Design review of the part shown in the three views and the two pictorial views. Dimensions are in mm from the part's minimum x, y and z. Give positions to 0.01 mm unless a question says otherwise; leave off trailing zeros. Order: outer loops, then holes, each group sorted by start corner. A loop starts at its lowest first (then second) coordinate and runs counter-clockwise, first axis right, second up. Notation, with made-up numbers: (8.5, -24.75) - (65.5, -24.75) arc R29 ccw to (65.5, 7.25) - close; hole circle Ø6 at (22.25, -3). An arc over 180 degrees is marked (long way). Put each result on its own line as item: value. Start each with the question number.
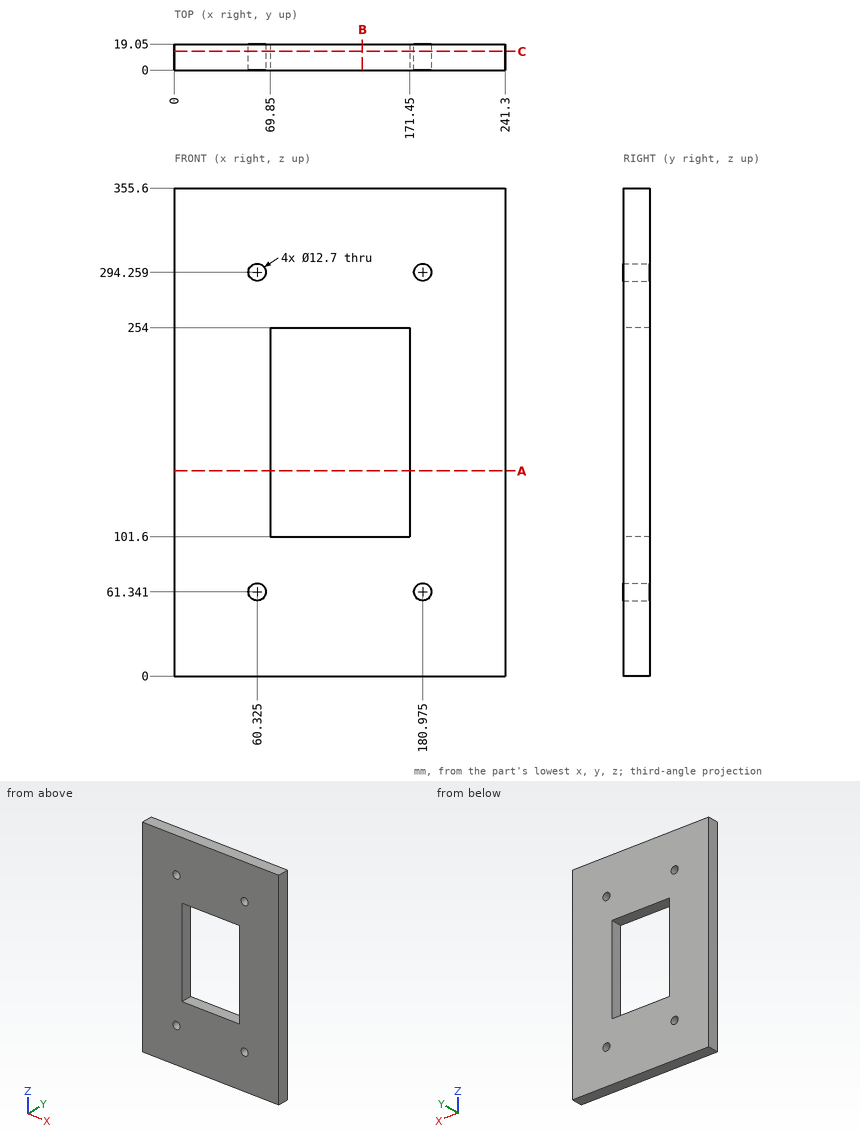
1. Add section A-A, the plane z = 149.5. Give the boundary of the cut face in (x, y).
2. Add section B-B, the plane x = 137. Give the boundary of the cut face in (y, z), then the cut area to 3 significant figures.
3. Add section C-C, the plane y = 13.75. Give the boundary of the cut face in (x, z) (3 decimals).
4. Wall thickness on line 1 (Z direction, x = 97, y = 14.5); line 2 (Z direction, x = 180, y = 12.5); line 3 (X direction, y = 7.25, z = 212.5): over which ranges is each line inside the solid? List them lowest first. Write a range as from..to.
Found:
1. outline: (0, 0) - (69.85, 0) - (69.85, 19.05) - (0, 19.05) - close; (171.45, 0) - (241.3, 0) - (241.3, 19.05) - (171.45, 19.05) - close
2. outline: (0, 0) - (19.05, 0) - (19.05, 101.6) - (0, 101.6) - close; (0, 254) - (19.05, 254) - (19.05, 355.6) - (0, 355.6) - close
2. area: 3,870 mm^2
3. outline: (0, 0) - (241.3, 0) - (241.3, 355.6) - (0, 355.6) - close; hole circle Ø12.7 at (60.325, 61.341); hole circle Ø12.7 at (60.325, 294.259); hole (69.85, 101.6) - (171.45, 101.6) - (171.45, 254) - (69.85, 254) - close; hole circle Ø12.7 at (180.975, 61.341); hole circle Ø12.7 at (180.975, 294.259)
4. line 1: z = 0..101.6, 254..355.6
4. line 2: z = 0..55.07, 67.62..287.98, 300.53..355.6
4. line 3: x = 0..69.85, 171.45..241.3
